Work out the finished part from the listing and answer in its coordinate system (mm). A direction names the side the tool comes from. Give positions to 0.01 mm unless a question says otherwise; leave off trailing zeros. Loops run counter-clockwise (first coordinate to the right, second up) from the corner with the lowest first, then second, coordinate; pieces in that order, holes last.
```python
from build123d import *

# Parameters (mm, degrees)
F3_DEPTH      = 32.001
F3_DEPTH_BACK = 32.001
F5_DEPTH      = 32.001
F5_DEPTH_BACK = 32.001


# Not quite as in the source:
# - a feature names something its author has since deleted; it is built from what else it names


with BuildPart() as f1:
    # F0 (on Top) → F1 (revolve)
    with BuildSketch(Plane.XY):
        with BuildLine():
            Line((29, 3), (0, 3))
            Line((0, 3), (0, 0))
            Line((0, 0), (20.7, 0))
            ThreePointArc((20.7, 0), (22.1142135624, -0.5857864376), (22.7, -2))
            Line((22.7, -2), (22.7, -7.2844397868))
            ThreePointArc((22.7, -7.2844397868), (22.7497180358, -7.4498451628), (22.8823929227, -7.5604263361))
            ThreePointArc((22.8823929227, -7.5604263361), (23.3097624273, -7.6192211516), (23.7078530386, -7.45301228))
            Line((23.7078530386, -7.45301228), (27.5, -4.5))
            Line((27.5, -4.5), (24.5, -5.4))
            Line((24.5, -5.4), (24.5, -3))
            Line((24.5, -3), (24.5, 0))
            Line((24.5, 0), (32, 0))
            Line((32, 0), (29, 3))
        make_face()
    revolve(axis=Axis((0, -3.2623065636, 0), (0, -1, 0)))

    # F2 (on Top) → F3 (cut, two sides)
    with BuildSketch(Plane.XY) as f3_sk:
        with BuildLine():
            Line((-4, 0), (-18, 0))
            ThreePointArc((-18, 0), (-20.8284271247, -1.1715728753), (-22, -4))
            Line((-22, -4), (-22, -24.4516061772))
            Line((-22, -24.4516061772), (-4, -24.4516061772))
            Line((-4, -24.4516061772), (-4, 0))
        make_face()
        with BuildLine():
            Line((18, 0), (4, 0))
            Line((4, 0), (4, -24.4516061772))
            Line((4, -24.4516061772), (22, -24.4516061772))
            Line((22, -24.4516061772), (22, -4))
            ThreePointArc((22, -4), (20.8284271247, -1.1715728753), (18, 0))
        make_face()
    extrude(amount=-F3_DEPTH, mode=Mode.SUBTRACT)
    extrude(f3_sk.sketch, amount=F3_DEPTH_BACK, mode=Mode.SUBTRACT)

    # F4 (on Right) → F5 (cut, two sides)
    with BuildSketch(Plane.YZ) as f5_sk:
        with BuildLine():
            Line((-9.7492614017, 4), (0, 4))
            Line((0, 4), (0, 18))
            ThreePointArc((0, 18), (-1.1715728753, 20.8284271247), (-4, 22))
            Line((-4, 22), (-9.7492614017, 22))
            Line((-9.7492614017, 22), (-9.7492614017, 4))
        make_face()
        with BuildLine():
            Line((0, -18), (0, -4))
            Line((0, -4), (-9.764377423, -4))
            Line((-9.764377423, -4), (-9.764377423, -22))
            Line((-9.764377423, -22), (-4, -22))
            ThreePointArc((-4, -22), (-1.1715728753, -20.8284271247), (0, -18))
        make_face()
    extrude(amount=-F5_DEPTH, mode=Mode.SUBTRACT)
    extrude(f5_sk.sketch, amount=F5_DEPTH_BACK, mode=Mode.SUBTRACT)


solid = f1.part
```
Q1. Section A-A on y = -1 is taken. Give the vertices of the cut face in (x, z).
Q2. Section C-C on z = 0 is taken. Give the vertices of the cut face in (x, y).
Q3. Section B-B on x = 0 is taken. Give the vertices of the cut face in (y, z).
Q4. Which of the six approach directions +Z, -Z, +X, -X, +Y, -Y give full straight-line access (tool end or side, diameter ignored) to faces 1 (the face through (4, -4, 23)), 2 (the face through (23, -4, -4)), 3 (the face through (0.1, -4.7, 22.7))?
Q5. Given pin 1 (1.5 mm diameter, centred on x = -22, z = 6, fed in from -Y); pin 2 (2 mm diameter, centred on x = -25.5, y = -5.5, fed in from +Z); pin 3 (5.5 mm diameter, centred on y = -4.5, z = 24, fed in from -X), each flat-ended and moving along its own axis, determine where each tip first touches the part or whether it passes through.
Q6. Consider line 1 along Y through (x, z) = (11, 25); line 2 along X through (y, z) = (-5.75, -24); line 3 along X through (y, z) = (-4.25, -3.5). Determine where each line is inside the solid, lowest interval first.
Q7. Determine the mould class of faces 4 (the face through (-3.79, 2.85, 28.9)), 5 (the face through (25.979, -4.956, -0.06)), 6 (the face through (-25.979, -4.956, 0.06)), 7 (the face through (-4, -4, 23)) for opening direction Z: +Z half, -Z half, draft (parallel to the pull), parting line (faces both ways), or undercut.
Check result:
1. outline: (-24.17, -4) - (-22.07, -4) arc R22.43 cw to (-22.07, 4) - (-24.17, 4) arc R24.5 ccw to start; (-4, -24.17) arc R24.5 ccw to (4, -24.17) - (4, -22.07) arc R22.43 cw to (-4, -22.07) - close; (-4, 22.07) arc R22.43 cw to (4, 22.07) - (4, 24.17) arc R24.5 ccw to (-4, 24.17) - close; (22.07, -4) - (24.17, -4) arc R24.5 ccw to (24.17, 4) - (22.07, 4) arc R22.43 cw to start
2. outline: (-32, 0) - (-24.5, 0) - (-24.5, -5.4) - (-27.5, -4.5) - (-23.71, -7.45) arc R0.82 ccw to (-22.88, -7.56) arc R0.3 ccw to (-22.7, -7.28) - (-22.7, -2) arc R2 cw to (-20.7, 0) - (20.7, 0) arc R2 cw to (22.7, -2) - (22.7, -7.28) arc R0.3 ccw to (22.88, -7.56) arc R0.82 ccw to (23.71, -7.45) - (27.5, -4.5) - (24.5, -5.4) - (24.5, 0) - (32, 0) - (29, 3) - (-29, 3) - close
3. outline: (-7.56, -22.88) arc R0.82 ccw to (-7.45, -23.71) - (-4.5, -27.5) - (-5.4, -24.5) - (0, -24.5) - (0, -32) - (3, -29) - (3, 29) - (0, 32) - (0, 24.5) - (-5.4, 24.5) - (-4.5, 27.5) - (-7.45, 23.71) arc R0.82 ccw to (-7.56, 22.88) arc R0.3 ccw to (-7.28, 22.7) - (-2, 22.7) arc R2 cw to (0, 20.7) - (0, -20.7) arc R2 cw to (-2, -22.7) - (-7.28, -22.7) arc R0.3 ccw to start
4. face 1: +Z, -Z, +X, -Y
4. face 2: -Z, +X, -X, -Y
4. face 3: -Y
5. pin 1: stops at y = 0
5. pin 2: stops at z = 4
5. pin 3: stops at x = -4
6. line 1: y = 0 to 3
6. line 2: x = -4 to 4
6. line 3: x = -24.25 to -22.43, 22.43 to 24.25
7. face 4: parting line
7. face 5: undercut
7. face 6: undercut
7. face 7: draft
